Can you work these out from the model? Positions are in its coordinate system, mm. Face numbers are marked on the shaded views. Coordinates: 2 decimals unless noted, no trailing zeros. Order: outer loops, then holes, each group sorted by start corner. A loop starts at its lowest first (then second) coordinate and runs counter-clockwise, first axis right, second up.
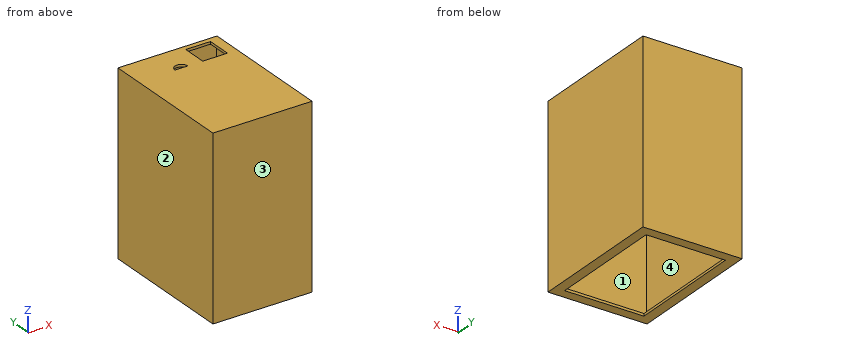
Autodesk Inventor part; units mm, degrees
ref_plane "YZ Plane" through (0, 0, 0) normal (1, 0, 0) x (0, 1, 0)
ref_plane "XZ Plane" through (0, 0, 0) normal (0, 1, 0) x (-1, 0, 0)
ref_plane "XY Plane" through (0, 0, 0) normal (0, 0, 1) x (1, 0, 0)
sketch "Sketch1" plane through (0, 0, 0) normal (0, 1, 0) x (-1, 0, 0)
  line L0 (0, 0) -> (127, 0)
  line L1 (127, 0) -> (127, -228.6)
  line L2 (127, -228.6) -> (0, -228.6)
  line L3 (0, -228.6) -> (0, 0)
  dimension "d0" = 127
  dimension "d1" = 228.6
extrude "Extrusion1" add sketch "Sketch1" along normal blind 177.8
sketch "Sketch2" plane through (0, 0, -228.6) normal (0, 0, -1) x (-1, 0, 0)
  line L0 (127, 0) -> (0, 0)
  line L1 (127, 0) -> (127, 177.8)
  line L2 (0, 177.8) -> (127, 177.8)
  line L3 (0, 0) -> (0, 177.8)
  line L4 (114.3, 165.1) -> (114.3, 12.7)
  line L5 (114.3, 12.7) -> (12.7, 12.7)
  line L6 (12.7, 12.7) -> (12.7, 165.1)
  line L7 (12.7, 165.1) -> (114.3, 165.1)
  dimension "d4" = 12.7
shell "Shell1" thickness 3.175 removed faces 1 at (-84.6667, 59.2667, -228.6)
extrude "Extrusion2" add sketch "Sketch2" against normal blind 3.175
sketch "Sketch3" plane through (-127, 0, 0) normal (0, 0, 1) x (1, 0, 0)
  line L0 (127, 0) -> (127, 177.8)
  line L1 (0, 177.8) -> (127, 177.8)
  line L2 (114.3, 171.45) -> (82.55, 171.45)
  line L3 (82.55, 171.45) -> (82.55, 139.7)
  line L4 (82.55, 139.7) -> (114.3, 139.7)
  line L5 (114.3, 139.7) -> (114.3, 171.45)
  dimension "d10" = 31.75
  dimension "d11" = 31.75
  dimension "d12" = 6.35
  dimension "d13" = 12.7
extrude "Extrusion3" cut sketch "Sketch3" against normal blind 25.4
sketch "Sketch4" plane through (-127, 0, 0) normal (0, 0, 1) x (1, 0, 0)
  line L0 (46.99, 139.7) -> (63.5, 139.7)
  line L1 (127, 0) -> (127, 177.8)
  arc A0 (63.5, 139.7) -> (46.99, 139.7) centre (55.245, 139.7) ccw
  dimension "d16" = 16.51
  dimension "d19" = 63.5
  dimension "d20" = 38.1
extrude "Extrusion4" cut sketch "Sketch4" against normal blind 25.4
properties part number "Electronics_Box"
1. Please list where these lines run through material, in increasing order: probe 1 along X at (y, z) = (21, -215.5) (3 decimals); probe 2 along Z at (x, y) = (-111, 10.5) (3 decimals); probe 3 along Y at (x, z) = (-88.5, -14.5) (3 decimals).
Completed:
probe 1: x = -127 to -123.825, -3.175 to 0
probe 2: z = -228.6 to -225.425, -3.175 to 0
probe 3: y = 0 to 3.175, 174.625 to 177.8
2. Imagine slicing it at C-C on z = -109.5. Please give me the cut outline in (x, y) (3 decimals).
Completed:
outline: (-127, 0) - (0, 0) - (0, 177.8) - (-127, 177.8) - close; hole (-123.825, 3.175) - (-3.175, 3.175) - (-3.175, 174.625) - (-123.825, 174.625) - close
3. Imagine slicing it at B-B on y = 79.5. Please give me the cut outline in (x, z) (3 decimals).
Completed:
outline: (-127, -228.6) - (-114.3, -228.6) - (-114.3, -225.425) - (-123.825, -225.425) - (-123.825, -3.175) - (-3.175, -3.175) - (-3.175, -225.425) - (-12.7, -225.425) - (-12.7, -228.6) - (0, -228.6) - (0, 0) - (-127, 0) - close
4. Imagine slicing it at D-D on x = -58. Please give me the cut outline in (y, z) (3 decimals), then the cut area to 3 significant figures.
Completed:
outline: (0, -228.6) - (12.7, -228.6) - (12.7, -225.425) - (3.175, -225.425) - (3.175, -3.175) - (174.625, -3.175) - (174.625, -225.425) - (165.1, -225.425) - (165.1, -228.6) - (177.8, -228.6) - (177.8, 0) - (0, 0) - close
area: 2,060 mm2
5. Thinking about a two-plate mould opening in X: for the marked faces 1, 2, 3 and 4, which applies, pulls with the +X half, pulls with the -X half, needs draft (parallel to the pull), parting line crosses it, or undercut?
Completed:
face 1: undercut
face 2: pulls with the -X half
face 3: needs draft
face 4: undercut
6. Imagine slicing it at A-A on x = -37.5. Please give me the cut outline in (y, z) (3 decimals).
Completed:
outline: (0, -228.6) - (12.7, -228.6) - (12.7, -225.425) - (3.175, -225.425) - (3.175, -3.175) - (139.7, -3.175) - (139.7, 0) - (0, 0) - close; (165.1, -228.6) - (177.8, -228.6) - (177.8, 0) - (171.45, 0) - (171.45, -3.175) - (174.625, -3.175) - (174.625, -225.425) - (165.1, -225.425) - close
